```python
from build123d import *

# Parameters (mm, degrees)
SKETCH1_W           = 600
SKETCH1_H           = 20
BOSS_EXTRUDE1_DEPTH = 270
CUT_EXTRUDE1_DEPTH  = 18
CUT_EXTRUDE2_DEPTH  = 2


with BuildPart() as part:
    # Sketch1 → Boss-Extrude1 (new body)
    with BuildSketch(Plane.XY):
        with Locations((221.099899989, 5.665003505)):
            Rectangle(SKETCH1_W, SKETCH1_H)
    extrude(amount=-BOSS_EXTRUDE1_DEPTH)

    # 3DSketch1 → Cut-Extrude1 (cut)
    with BuildSketch(Plane(origin=(519.099899989, 15.665003505, -268), x_dir=(-0.9131786164814929, 0, 0.4075595838659012), z_dir=(0, 1, 0))):
        Polygon((0, 0), (544.254455423, -242.905511984), (652.665304731, 0), (108.410849308, 242.905511984), align=None)
    extrude(amount=-CUT_EXTRUDE1_DEPTH, mode=Mode.SUBTRACT)

    # 3DSketch2 → Cut-Extrude2 (cut)
    with BuildSketch(Plane(origin=(-58.900100011, -2.334996495, -250), x_dir=(0.9250198183784529, 0, 0.3799188539768646), z_dir=(0, 1, 0))):
        Polygon((0, 0), (518.011098292, 212.754558227), (605.392434707, 0), (87.381336415, -212.754558227), align=None)
    extrude(amount=-CUT_EXTRUDE2_DEPTH, mode=Mode.SUBTRACT)


solid = part.part
```
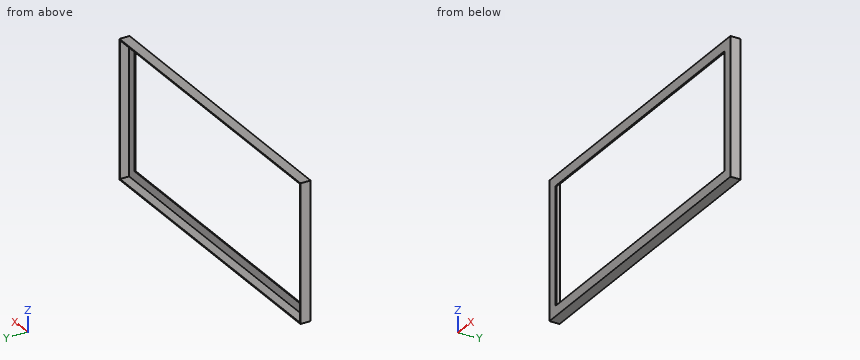
Model file for the job. Use its own axes, mm. Round coordinates to 2 decimals unless told otherwise and drop trailing zeros. Write each loop counter-clockwise with the first axis right and the second up, starting at its lowest first coordinate (ties: lowest second). Pieces come first, ordered by that corner, then holes. Notation, with made-up numbers: (9.25, 76.5) -> (27.25, 76.5) arc R7 ccw to (27.25, 82.5) -> close; hole circle Ø10 at (65, -12). An arc over 180 degrees is marked (long way). Answer as CSV lines item,"result".
1. Slice it at A-A, the plane x = 42. List the corners of the cut face in (y, z) (3 decimals), plus the area to 3 significant figures.
Resolved:
outline,"(-4.335, -270) -> (15.665, -270) -> (15.665, -268) -> (-2.335, -268) -> (-2.335, -250) -> (-4.335, -250) -> close; (-4.335, -20) -> (-2.335, -20) -> (-2.335, -2) -> (15.665, -2) -> (15.665, 0) -> (-4.335, 0) -> close"
area,"152 mm²"
2. Slice it at B-B, the plane z = -125. List the corners of the cut face in (x, y) (3 decimals).
Resolved:
outline,"(-78.9, -4.335) -> (-58.9, -4.335) -> (-58.9, -2.335) -> (-76.9, -2.335) -> (-76.9, 15.665) -> (-78.9, 15.665) -> close; (501.1, -4.335) -> (521.1, -4.335) -> (521.1, 15.665) -> (519.1, 15.665) -> (519.1, -2.335) -> (501.1, -2.335) -> close"
3. Slice it at C-C, the plane y = 7.25. List the corners of the cut face in (x, z).
Resolved:
outline,"(-78.9, -270) -> (521.1, -270) -> (521.1, 0) -> (-78.9, 0) -> close; hole (-76.9, -268) -> (519.1, -268) -> (519.1, -2) -> (-76.9, -2) -> close"
4. Drill centre lines: line 1 (X direction, y = 9.75, z = -257); line 2 (X direction, y = -3.5, z = -134); line 3 (Z direction, x = 76, y = -2.75). Where is each one in solid material? Low to high.
Resolved:
line 1,"-78.9 to -76.9, 519.1 to 521.1"
line 2,"-78.9 to -58.9, 501.1 to 521.1"
line 3,"-270 to -250, -20 to 0"
